```python
from build123d import *

# Parameters (mm, degrees)
F0_W         = 78
F0_H         = 78
F1_DEPTH     = 61
F2_T         = -4
F3_W         = 74
F3_H         = 74
F3_W_2       = 70
F3_H_2       = 70
F4_DEPTH     = 20
F6_DEPTH     = 2
F7_R         = 4
F8_R         = 4
F9_W         = 40
F9_H         = 2
F10_DEPTH    = 0.3
F11_T1_DEPTH = 43.5707142143


# Not quite as in the source:
# - a fillet or chamfer that OpenCascade refuses, or shapes differently, is made with other operations: its cross-section is extruded or revolved along the edge and cut away or added


with BuildPart() as f1:
    # F0 (on Top) → F1 (new body)
    with BuildSketch(Plane.XY):
        Rectangle(F0_W, F0_H)
    extrude(amount=F1_DEPTH)

    # F2
    f2_openings = [f1.faces().sort_by_distance(p)[0] for p in [
        (0, 0, 61),
    ]]
    offset(amount=F2_T, openings=f2_openings)

    # F3 (on face) → F4 (cut)
    with BuildSketch(Plane.XY.offset(61)):
        Rectangle(F3_W, F3_H)
        Rectangle(F3_W_2, F3_H_2, mode=Mode.SUBTRACT)
    extrude(amount=-F4_DEPTH, mode=Mode.SUBTRACT)

    # F5 (on face) → F6 (cut)
    with BuildSketch(Plane.XZ.offset(-37)):
        with BuildLine():
            Line((27, 61), (-27, 61))
            ThreePointArc((-27, 61), (0, 54), (27, 61))
        make_face()
    extrude(amount=-F6_DEPTH, mode=Mode.SUBTRACT)

    # F7
    f7_edges = [f1.edges().sort_by_distance(p)[0] for p in [
        (-39, 39, 30.5),
        (39, 39, 30.5),
        (39, -39, 30.5),
        (-39, -39, 30.5),
        (-39, 0, 0),
        (0, -39, 0),
        (39, 0, 0),
        (0, 39, 0),
    ]]
    fillet(f7_edges, radius=F7_R)

    # F8
    f8_edges = [f1.edges().sort_by_distance(p)[0] for p in [
        (37, -37, 51),
        (-37, -37, 51),
        (37, 37, 51),
        (-37, 37, 51),
    ]]
    fillet(f8_edges, radius=F8_R)

    # F9 (on face) → F10 (cut)
    with BuildSketch(Plane.YZ.offset(-37)):
        with Locations((0, 51)):
            Rectangle(F9_W, F9_H)
    extrude(amount=-F10_DEPTH, mode=Mode.SUBTRACT)

    # F11: fillet of radius 1 on 2 edges, made by hand

    # F11_s2 → F11_t1 (join)
    with BuildSketch(Plane.XZ.offset(-21.7853571071)):
        with BuildLine():
            ThreePointArc((-37, 50), (-37.2219544457, 50.3268445082), (-37.3, 50.7141428429))
            Line((-37.3, 50.7141428429), (-37.3, 50))
            Line((-37.3, 50), (-37, 50))
        make_face()
        with BuildLine():
            ThreePointArc((-37, 52), (-37.2219544457, 51.6731554918), (-37.3, 51.2858571571))
            Line((-37.3, 51.2858571571), (-37.3, 52))
            Line((-37.3, 52), (-37, 52))
        make_face()
    extrude(amount=F11_T1_DEPTH)


solid = f1.part
```
Source: CAD feature listing. Evaluate the final solid. Frame: model axes, mm. A direction names the side the tool comes from. Round coordinates to 2 decimals unless told otherwise and drop trailing zeros. Order: outer loops, then holes, each group sorted by start corner. A loop starts at its lowest first (then second) coordinate and runs counter-clockwise, first axis right, second up. Notation, with made-up numbers: (-27, 35) -> (-18, 35) arc R20 ccw to (-18, 42) -> close; hole circle Ø3 at (62.5, 59.25). An arc over 180 degrees is marked (long way). Use CSV: the item, a comma, the result in double quotes.
(1) Access query for faces 1 (the face through (-39, 0, 32)), 2 (the face through (37, 0, 51)). Directions: +Z, -Z, +X, -X, +Y, -Y. A direction counts if a zero-diameter tool reaches every point of the face in a straight line with its end or side. Return the directions, or none.
Report:
face 1,"+Z, -Z, -X, +Y, -Y"
face 2,"+Z"
(2) Section C-C on x = 7. Return the cut outline in (y, z), and give its area (3 significant figures).
Report:
outline,"(-39, 4) arc R4 ccw to (-35, 0) -> (35, 0) arc R4 ccw to (39, 4) -> (39, 54.44) -> (37, 54.44) -> (37, 41) -> (35, 41) -> (35, 4) -> (-35, 4) -> (-35, 41) -> (-37, 41) -> (-37, 61) -> (-39, 61) -> close"
area,"668 mm^2"
(3) Section A-A on z = 26. Return the cut outline in (x, y).
Report:
outline,"(-39, -35) arc R4 ccw to (-35, -39) -> (35, -39) arc R4 ccw to (39, -35) -> (39, 35) arc R4 ccw to (35, 39) -> (-35, 39) arc R4 ccw to (-39, 35) -> close; hole (-35, -35) -> (35, -35) -> (35, 35) -> (-35, 35) -> close"
(4) Ray query, L1, parallel to X at y = 18.5, z = 21; L2, parallel to X at y = 16.5, z = 57. Return the intervals inside material, ascending.
Report:
L1,"-39 to -35, 35 to 39"
L2,"-39 to -37, 37 to 39"
(5) Section D-D on y = -5. Return the cut outline in (x, z).
Report:
outline,"(-39, 4) arc R4 ccw to (-35, 0) -> (35, 0) arc R4 ccw to (39, 4) -> (39, 61) -> (37, 61) -> (37, 41) -> (35, 41) -> (35, 4) -> (-35, 4) -> (-35, 41) -> (-37, 41) -> (-37, 50) arc R1 cw to (-37.3, 50.71) -> (-37.3, 51.29) arc R1 cw to (-37, 52) -> (-37, 61) -> (-39, 61) -> close"
(6) Section B-B on y = -31.5. Return the cut outline in (x, z), and give its area (3 significant figures).
Report:
outline,"(-39, 4) arc R4 ccw to (-35, 0) -> (35, 0) arc R4 ccw to (39, 4) -> (39, 61) -> (37, 61) -> (37, 41) -> (35, 41) -> (35, 4) -> (-35, 4) -> (-35, 41) -> (-37, 41) -> (-37, 61) -> (-39, 61) -> close"
area,"681 mm^2"
(7) First-contact query: pin 1 Ø21 at (x, y) = (-17.5, -7) entering from +Z. Flat tip, straight axial feed; report the tip coordinate or a pass-through.
Report:
pin 1,"z = 4"
(8) Pull-direction query (X, two-part tool) for faces 3 (the face through (35.797, -35.859, 50.86)), 4 (the face through (39, 0, 32)), 5 (the face through (-35.797, 35.859, 50.86)), 6 (the face through (-37.859, 0.49, 1.203)); classes: +X half, -X half, draft (parallel to the pull), parting line (faces both ways), or undercut.
Report:
face 3,"undercut"
face 4,"+X half"
face 5,"undercut"
face 6,"-X half"
